from build123d import *

# Parameters (mm, degrees)
SKIZZE1_W                       = 330
SKIZZE1_H                       = 156
AUFSATZ_LINEAR_AUSTRAGEN1_DEPTH = 4
SKIZZE2_R                       = 2.25
SKIZZE2_W                       = 31.1
SKIZZE2_H                       = 110
SCHNITT_LINEAR_AUSTRAGEN1_DEPTH = 183.551362635
M3_GEWINDEBOHRUNG1_D            = 2.5
SKIZZE5_R                       = 19
SCHNITT_LINEAR_AUSTRAGEN2_DEPTH = 183.551362635
VERRUNDUNG1_R                   = 2
SKIZZE7_R                       = 1.6
SKIZZE7_W                       = 11.7
SKIZZE7_H                       = 18.6
SCHNITT_LINEAR_AUSTRAGEN3_DEPTH = 183.551362635
SCHNITT_LINEAR_AUSTRAGEN4_DEPTH = 183.551362635
VERRUNDUNG2_R                   = 2
SKIZZE10_W                      = 4
SKIZZE10_H                      = 30
SCHNITT_LINEAR_AUSTRAGEN5_DEPTH = 183.551362635


with BuildPart() as part:
    # Skizze1 → Aufsatz-Linear austragen1 (new body)
    with BuildSketch(Plane.XY):
        Rectangle(SKIZZE1_W, SKIZZE1_H)
    extrude(amount=AUFSATZ_LINEAR_AUSTRAGEN1_DEPTH)

    # Skizze2 → Schnitt-Linear austragen1 (cut, through all)
    with BuildSketch(Plane.XY.offset(4)):
        with Locations((-105.9, 46)):
            Circle(SKIZZE2_R)
        with Locations((-105.9, -46)):
            Circle(SKIZZE2_R)
        with Locations((105.9, -46)):
            Circle(SKIZZE2_R)
        with Locations((105.9, 46)):
            Circle(SKIZZE2_R)
        with Locations((-40, 65)):
            Circle(SKIZZE2_R)
        with Locations((40, 65)):
            Circle(SKIZZE2_R)
        with Locations((-40, -65)):
            Circle(SKIZZE2_R)
        with Locations((40, -65)):
            Circle(SKIZZE2_R)
        with Locations((-135, -65)):
            Circle(SKIZZE2_R)
        with Locations((-135, 65)):
            Circle(SKIZZE2_R)
        with Locations(Location((135, -65, 0), (0, 0, 180))):
            Circle(SKIZZE2_R)
        with Locations(Location((135, 65, 0), (0, 0, 180))):
            Circle(SKIZZE2_R)
        with Locations((133.45, 0)):
            Rectangle(SKIZZE2_W, SKIZZE2_H)
        with Locations((-133.45, 0)):
            Rectangle(SKIZZE2_W, SKIZZE2_H)
    extrude(amount=-SCHNITT_LINEAR_AUSTRAGEN1_DEPTH, mode=Mode.SUBTRACT)

    # M3 Gewindebohrung1 (through all)
    with Locations(Plane.XY.offset(4)):
        with Locations((16, -16), (0, 0), (16, 16), (-16, -16), (-16, 16)):
            Hole(M3_GEWINDEBOHRUNG1_D / 2)

    # Skizze5 → Schnitt-Linear austragen2 (cut, through all)
    with BuildSketch(Plane.XY.offset(4)):
        Circle(SKIZZE5_R)
    extrude(amount=-SCHNITT_LINEAR_AUSTRAGEN2_DEPTH, mode=Mode.SUBTRACT)

    # Verrundung1
    verrundung1_edges = [part.edges().sort_by_distance(p)[0] for p in [
        (149, 55, 2),
        (149, -55, 2),
        (117.9, -55, 2),
        (117.9, 55, 2),
        (-149, -55, 2),
        (-149, 55, 2),
        (-117.9, 55, 2),
        (-117.9, -55, 2),
    ]]
    fillet(verrundung1_edges, radius=VERRUNDUNG1_R)

    # Skizze7 → Schnitt-Linear austragen3 (cut, through all)
    with BuildSketch(Plane.XY.offset(4)):
        with Locations((-12, -27.880186595)):
            Circle(SKIZZE7_R)
        with Locations((-12, -53.280186595)):
            Circle(SKIZZE7_R)
        with Locations(Location((12, -53.280186595, 0), (0, 0, 180))):
            Circle(SKIZZE7_R)
        with Locations(Location((12, -27.880186595, 0), (0, 0, 180))):
            Circle(SKIZZE7_R)
        with BuildLine():
            Line((-6.8, 46.612478374), (-6.8, 39.387521626))
            ThreePointArc((-6.8, 39.387521626), (0, 35.3), (6.8, 39.387521626))
            Line((6.8, 39.387521626), (6.8, 46.612478374))
            ThreePointArc((6.8, 46.612478374), (0, 50.7), (-6.8, 46.612478374))
        make_face()
        with Locations((-12, -40.580186595)):
            Rectangle(SKIZZE7_W, SKIZZE7_H)
        with Locations((12, -40.580186595)):
            Rectangle(SKIZZE7_W, SKIZZE7_H)
    extrude(amount=-SCHNITT_LINEAR_AUSTRAGEN3_DEPTH, mode=Mode.SUBTRACT)

    # Skizze9 → Schnitt-Linear austragen4 (cut, through all)
    with BuildSketch(Plane.XY.offset(4)):
        Polygon((53.9, 55), (53.9, 7), (53.9, -7), (53.9, -55), (93.9, -55), (93.9, -7), (93.9, 7), (93.9, 55), align=None)
        Polygon((53.9, 55), (53.9, 7), (53.9, -7), (53.9, -55), (93.9, -55), (93.9, -7), (93.9, 7), (93.9, 55), align=None)
        Polygon((-53.9, 7), (-53.9, -7), (-53.9, -55), (-93.9, -55), (-93.9, -7), (-93.9, 7), (-93.9, 55), (-53.9, 55), align=None)
    extrude(amount=-SCHNITT_LINEAR_AUSTRAGEN4_DEPTH, mode=Mode.SUBTRACT)

    # Verrundung2
    verrundung2_edges = [part.edges().sort_by_distance(p)[0] for p in [
        (93.9, 55, 2),
        (93.9, -55, 2),
        (53.9, -55, 2),
        (53.9, 55, 2),
        (-53.9, 55, 2),
        (-53.9, -55, 2),
        (-93.9, -55, 2),
        (-93.9, 55, 2),
    ]]
    fillet(verrundung2_edges, radius=VERRUNDUNG2_R)

    # Skizze10 → Schnitt-Linear austragen5 (cut, through all)
    with BuildSketch(Plane.XY.offset(4)):
        with Locations((-28, 31)):
            Rectangle(SKIZZE10_W, SKIZZE10_H)
        with Locations((-28, -31)):
            Rectangle(SKIZZE10_W, SKIZZE10_H)
        with Locations((28, -31)):
            Rectangle(SKIZZE10_W, SKIZZE10_H)
        with Locations((28, 31)):
            Rectangle(SKIZZE10_W, SKIZZE10_H)
        with Locations((-163, -31)):
            Rectangle(SKIZZE10_W, SKIZZE10_H)
        with Locations((-163, 31)):
            Rectangle(SKIZZE10_W, SKIZZE10_H)
        with Locations((163, -31)):
            Rectangle(SKIZZE10_W, SKIZZE10_H)
        with Locations((163, 31)):
            Rectangle(SKIZZE10_W, SKIZZE10_H)
    extrude(amount=-SCHNITT_LINEAR_AUSTRAGEN5_DEPTH, mode=Mode.SUBTRACT)


solid = part.part
Verification items for the finished model (mm, model axes). Coordinates: 2 decimals unless noted, no trailing zeros. Loops run counter-clockwise (first coordinate to the right, second up) from the corner with the lowest first, then second, coordinate; pieces in that order, holes last. Notation, with made-up numbers: M 29,58 L 64,58 A9 ccw 64,62 Z; hole C -33,-24.5 d9. An arc over 180 degrees is marked long. One line per item, written item: value.
1. Section check B-B on z = 0.6. Give the number of separate pieces and of enclosed holes in the cut face, plus the area to 3 significant figures.
Answers follow:
separate pieces: 1
enclosed holes: 32
area: 32,900 mm^2
2. Gauge pin test, flat ends, axial feed: P1, Ø2, axis at y = 32, z = 2, coming from the -X side; P2, Ø2, axis at y = 37.5, z = 1.5, coming from the +X side. Record the tip position at first contact, or that the pin passes through.
Answers follow:
P1: x = -161
P2: x = 161
3. Mould release check, pull along X, two halves, no side actions. Record for faces 1 (the cylindrical face through (8.767, -16.856, 2.028)), 2 (the flat face through (-2, -34, 4)): pulls with the +X half, pulls with the -X half, needs draft (parallel to the pull), parting line crosses it, or undercut.
Answers follow:
face 1: undercut
face 2: needs draft
4. Material ranges on line 1 along Y through (x, z) = (-135, 2.6); line 2 along X through (y, z) = (1, 3.3); line 3 along Y through (x, z) = (-105.5, 1.4), recorded low to high. Write a range as from..to.
Answers follow:
line 1: -78..-67.25, -62.75..-55, 55..62.75, 67.25..78
line 2: -165..-149, -117.9..-93.9, -53.9..-18.97, 18.97..53.9, 93.9..117.9, 149..165
line 3: -78..-48.21, -43.79..43.79, 48.21..78
5. Section check A-A on x = 64.5. Record the cut outline in (y, z), plus the area to 3 significant figures.
Answers follow:
outline: M -78,0 L -55,0 L -55,4 L -78,4 Z; M 55,0 L 78,0 L 78,4 L 55,4 Z
area: 184 mm^2
